```python
from build123d import *

# Parameters (mm, degrees)
SKETCH2_W           = 50
SKETCH2_H           = 50
SKETCH2_W_2         = 40
SKETCH2_H_2         = 40
BOSS_EXTRUDE1_DEPTH = 150
CUT_EXTRUDE1_DEPTH  = 161.078105936
CUT_EXTRUDE2_DEPTH  = 161.078105936


with BuildPart() as part:
    # Sketch2 → Boss-Extrude1 (new body)
    with BuildSketch(Plane(origin=(0, 0, 0), x_dir=(1, 0, 0), z_dir=(0, 0, -1))):
        Rectangle(SKETCH2_W, SKETCH2_H)
        Rectangle(SKETCH2_W_2, SKETCH2_H_2, mode=Mode.SUBTRACT)
    extrude(amount=-BOSS_EXTRUDE1_DEPTH)

    # Sketch3 → Cut-Extrude1 (cut, through all)
    with BuildSketch(Plane.XZ.offset(25)):
        Polygon((0, 150), (25, 125), (25, 150), align=None)
    extrude(amount=-CUT_EXTRUDE1_DEPTH, mode=Mode.SUBTRACT)

    # Sketch4 → Cut-Extrude2 (cut, through all)
    with BuildSketch(Plane.XZ.offset(25)):
        Polygon((25, 0), (-25, 28.867513459), (-25, 0), align=None)
    extrude(amount=-CUT_EXTRUDE2_DEPTH, mode=Mode.SUBTRACT)


solid = part.part
```
Build history of the part. All positions in model axes, mm. A direction names the side the tool comes from. Round coordinates to 2 decimals unless told otherwise and drop trailing zeros. Loops run counter-clockwise (first coordinate to the right, second up) from the corner with the lowest first, then second, coordinate; pieces in that order, holes last.
Item 1: Which spindle directions (+Z, -Z, +X, -X, +Y, -Y) get a long thin tool onto all of the face, cutting with end or side? Do faces 1 (the face through (0, 25, 74)), 2 (the face through (20, 0, 66)). Say none if no direction does.
Item 2: Saw through at B-B (x = 7). List the corners of the cut face in (y, z).
Item 3: Saw through at A-A (y = 13). List the corners of the cut face in (x, z), then the cut area to 3 significant figures.
Item 4: Saw through at D-D (x = -21.5). List the corners of the cut face in (y, z), then the cut area to 3 significant figures.
Item 5: Drill centre lines: line 1 along X through (y, z) = (18, 39); line 2 along X through (y, z) = (14, 12). Where is each one in solid material? Low to high.
Item 6: Two-plate mould, pull along X, no slides. Class faces 3 (the face through (-25, 0, 89)), 4 (the face through (25, 0, 62)), 5 (the face through (0, 20, 75)): released by +X, released by -X, zero draft, split by the parting line, or undercut.
Item 7: Saw through at C-C (z = 34). List the corners of the cut face in (x, y).
Worked answers:
1. face 1: +Z, -Z, +X, -X, +Y
1. face 2: +Z, -Z
2. outline: (-25, 10.39) - (-20, 10.39) - (-20, 143) - (-25, 143) - close; (20, 10.39) - (25, 10.39) - (25, 143) - (20, 143) - close
3. outline: (-25, 28.87) - (-20, 25.98) - (-20, 150) - (-25, 150) - close; (20, 2.89) - (25, 0) - (25, 125) - (20, 130) - close
3. area: 1,240 mm2
4. outline: (-25, 26.85) - (25, 26.85) - (25, 150) - (-25, 150) - close
4. area: 6,160 mm2
5. line 1: x = -25 to -20, 20 to 25
5. line 2: x = 20 to 25
6. face 3: released by -X
6. face 4: released by +X
6. face 5: undercut
7. outline: (-25, -25) - (25, -25) - (25, 25) - (-25, 25) - close; hole (-20, -20) - (20, -20) - (20, 20) - (-20, 20) - close
